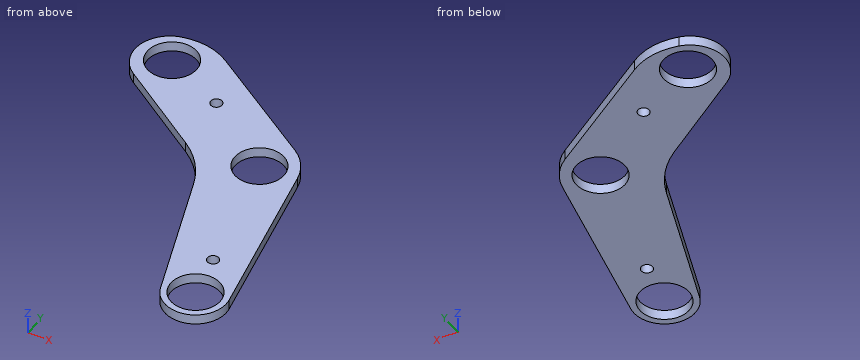
```python
from build123d import *

# Parameters (mm, degrees)
SKETCH1_R           = 14.2875
SKETCH1_R_2         = 3.302
BOSS_EXTRUDE1_DEPTH = 5.842
FILLET6_R           = 35.56
FILLET10_R          = 27.94
FILLET13_R          = 50.8
FILLET16_R          = 20.32


with BuildPart() as part:
    # Sketch1 → Boss-Extrude1 (new body)
    with BuildSketch(Plane(origin=(0, 0, 0), x_dir=(-1, 0, 0), z_dir=(0, 0, -1))):
        with BuildLine():
            Line((165.785053206, 142.946766421), (130.990896358, 174.574150067))
            Line((130.990896358, 174.574150067), (31.981087973, 112.057039535))
            Line((31.981087973, 112.057039535), (9.409224511, 1.710371233))
            ThreePointArc((9.409224511, 1.710371233), (21.197749586, -18.801775256), (43.01064713, -9.641263383))
            Line((43.01064713, -9.641263383), (77.484953862, 85.860414024))
            Line((77.484953862, 85.860414024), (165.785053206, 142.946766421))
        make_face()
        with Locations((130.990896358, 146.510317071)):
            Circle(SKETCH1_R, mode=Mode.SUBTRACT)
        with Locations((32.554001794, 24.213373462)):
            Circle(SKETCH1_R_2, mode=Mode.SUBTRACT)
        with Locations((94.707078764, 129.476886965)):
            Circle(SKETCH1_R_2, mode=Mode.SUBTRACT)
        with Locations((50.8, 98.679)):
            Circle(SKETCH1_R, mode=Mode.SUBTRACT)
        with Locations((26.917500437, -1.871018398)):
            Circle(SKETCH1_R, mode=Mode.SUBTRACT)
    extrude(amount=-BOSS_EXTRUDE1_DEPTH)

    # Fillet6
    fillet6_edges = [part.edges().sort_by_distance(p)[0] for p in [
        (-130.990896358, 174.574150067, 2.921),
    ]]
    fillet(fillet6_edges, radius=FILLET6_R)

    # Fillet10
    fillet10_edges = [part.edges().sort_by_distance(p)[0] for p in [
        (-31.981087973, 112.057039535, 2.921),
    ]]
    fillet(fillet10_edges, radius=FILLET10_R)

    # Fillet13
    fillet13_edges = [part.edges().sort_by_distance(p)[0] for p in [
        (-77.484953862, 85.860414024, 2.921),
    ]]
    fillet(fillet13_edges, radius=FILLET13_R)

    # Fillet16
    fillet16_edges = [part.edges().sort_by_distance(p)[0] for p in [
        (-165.785053206, 142.946766421, 2.921),
    ]]
    fillet(fillet16_edges, radius=FILLET16_R)


solid = part.part
```
Geometry check sheet. Reference: the model listing, model coordinates, mm. Give positions to 0.01 mm unless a question says otherwise; leave off trailing zeros. Loops run counter-clockwise (first coordinate to the right, second up) from the corner with the lowest first, then second, coordinate; pieces in that order, holes last. Notation, with made-up numbers: M 61,29 L 83,29 A15 ccw 83,35 Z; hole C 23.5,-7 d11. An arc over 180 degrees is marked long. Answer as CSV lines item,"result".
Item 1: Material ranges on line 1 (Y direction, x = -34, z = 4.5); line 2 (X direction, y = 22, z = 3.1); line 3 (Y direction, x = -141, z = 1.35), recorded low to high.
Values:
line 1,"y = -18.28 to -14.28, 10.54 to 21.24, 27.18 to 110.7"
line 2,"x = -54.43 to -35, -30.1 to -13.56"
line 3,"y = 126.92 to 136.31, 156.71 to 162.52"
Item 2: Cross-section at C-C on y = 64.5. Record the cut outline in (x, z), and give its area (3 significant figures).
Values:
outline,"M -69.77,0 L -22.25,0 L -22.25,5.84 L -69.77,5.84 Z"
area,"278 mm²"
Item 3: Cross-section at A-A on x = -47.5. Record the cut outline in (y, z), and give its area (3 significant figures).
Values:
outline,"M 2.8,0 L 84.78,0 L 84.78,5.84 L 2.8,5.84 Z; M 112.58,0 L 121.86,0 L 121.86,5.84 L 112.58,5.84 Z"
area,"533 mm²"
Item 4: Depth check by flat-ended pin: P1, Ø1, axis at y = 119.5, z = 1.5, coming from the +X side; P2, Ø12, axis at x = -45, y = 121.5, coming from the +Z side; P3, Ø2, axis at y = 75, z = 2.5, coming from the -X side; P4, Ø1, axis at y = 29.5, z = 4, coming from the -X side. Enter the tip coordinate at first touch or a pass-through.
Values:
P1,"stops at x = -42.98"
P2,"stops at z = 5.84"
P3,"stops at x = -74.41"
P4,"stops at x = -57.32"
Item 5: Cross-section at D-D on x = -110. Record the cut outline in (y, z).
Values:
outline,"M 106.88,0 L 161.24,0 L 161.24,5.84 L 106.88,5.84 Z"
Item 6: Cross-section at B-B on z = 3. Count the separate pieces of the cut face and the enclosed holes in it, and give its area (3 significant figures).
Values:
separate pieces,"1"
enclosed holes,"5"
area,"7,810 mm²"
